```python
from build123d import *

# Parameters (mm, degrees)
EXTRUDE_1_DEPTH        = 10
EXTRUDE_2_DEPTH        = 13.2
SKETCH_3_R             = 2.8
EXTRUDE_3_DEPTH        = 20.1058285
EXTRUDE_3_DEPTH_BACK   = 4
SKETCH_4_R             = 2.8
EXTRUDE_4_DEPTH        = 20.1058285
EXTRUDE_4_DEPTH_BACK   = 4.1058285
SKETCH_5_R             = 2.8
EXTRUDE_5_DEPTH        = 20.1058285
EXTRUDE_5_DEPTH_BACK   = 4.1058285
HOLE_WIZARD_M4_1_D     = 3.3
HOLE_WIZARD_M4_1_DEPTH = 10.1
HOLE_WIZARD_M4_1_TIP   = 0.991420021


with BuildPart() as part:
    # Sketch 1 → Extrude 1 (new body)
    with BuildSketch(Plane.XY):
        Polygon((0, -36.405628463), (31.572352781, 18.279290669), (-31.572352781, 18.279290669), align=None)
    extrude(amount=EXTRUDE_1_DEPTH)

    # Sketch 1_5 → Extrude 2 (add)
    with BuildSketch(Plane.XY):
        Polygon((11.960518161, 2.321180547), (14.039474758, 1.120894396), (16.117440099, -0.078819453), (18.517440099, 4.078102485), (14.360518161, 6.478102485), align=None)
        Polygon((-7.990460401, 9.197522296), (-7.990460401, 12.000572743), (-7.990460401, 13.997522296), (-12.790460401, 13.997522296), (-12.790460401, 9.197522296), align=None)
        Polygon((7.990460401, 14.002477704), (7.990460401, 12.004383545), (7.990460401, 9.202477704), (12.790460401, 9.202477704), (12.790460401, 14.002477704), align=None)
        Polygon((8.131271207, -13.921180547), (6.052314609, -12.720894396), (3.974349269, -11.521180547), (1.574349269, -15.678102485), (5.731271207, -18.078102485), align=None)
        Polygon((-3.97005776, -11.518702843), (-6.395424519, -12.918988994), (-8.126979698, -13.918702843), (-5.726979698, -18.075624781), (-1.57005776, -15.675624781), align=None)
        Polygon((-18.521731608, 4.075624781), (-16.121731608, -0.081297157), (-14.389185172, 0.918988994), (-11.96480967, 2.318702843), (-14.36480967, 6.475624781), align=None)
    extrude(amount=-EXTRUDE_2_DEPTH)

    # Sketch 3 → Extrude 3 (add, two sides)
    with BuildSketch(Plane(origin=(3.9952302, -6.919941695, 0), x_dir=(0.866025404, 0.5, 0), z_dir=(-0.5, 0.866025404, 0))) as extrude_3_sk:
        with Locations((-11.602477704, 13.2)):
            Circle(SKETCH_3_R)
    extrude(amount=EXTRUDE_3_DEPTH)
    extrude(extrude_3_sk.sketch, amount=-EXTRUDE_3_DEPTH_BACK)

    # Sketch 4 → Extrude 4 (add, two sides)
    with BuildSketch(Plane(origin=(-7.990460401, 0, 0), x_dir=(0, 0, -1), z_dir=(1, 0, 0))) as extrude_4_sk:
        with Locations((13.2, 11.602477704)):
            Circle(SKETCH_4_R)
    extrude(amount=EXTRUDE_4_DEPTH)
    extrude(extrude_4_sk.sketch, amount=-EXTRUDE_4_DEPTH_BACK)

    # Sketch 5 → Extrude 5 (add, two sides)
    with BuildSketch(Plane(origin=(3.9952302, 6.919941695, 0), x_dir=(-0.866025404, 0.5, 0), z_dir=(-0.5, -0.866025404, 0))) as extrude_5_sk:
        with Locations((-11.602477704, 13.2)):
            Circle(SKETCH_5_R)
    extrude(amount=EXTRUDE_5_DEPTH)
    extrude(extrude_5_sk.sketch, amount=-EXTRUDE_5_DEPTH_BACK)

    # Hole Wizard M4 _1
    with Locations(Plane.XY.offset(10)):
        with Locations((7.5, 5), (-7.5, 5)):
            Hole(HOLE_WIZARD_M4_1_D / 2, depth=HOLE_WIZARD_M4_1_DEPTH)
            with Locations((0, 0, -(HOLE_WIZARD_M4_1_DEPTH + HOLE_WIZARD_M4_1_TIP / 2))):  # 118° drill point
                Cone(0, HOLE_WIZARD_M4_1_D / 2, HOLE_WIZARD_M4_1_TIP, mode=Mode.SUBTRACT)


solid = part.part
```
Verification items for the finished model (mm, model axes). A direction names the side the tool comes from. Coordinates: 2 decimals unless noted, no trailing zeros. Write each loop counter-clockwise with the first axis right and the second up, starting at its lowest first coordinate (ties: lowest second). Pieces come first, ordered by that corner, then holes. Notation, with made-up numbers: M -3.75,-12.5 L 19.25,-12.5 A17 cw 19.25,12.5 Z; hole C 35.5,67.5 d6. An arc over 180 degrees is marked long. Answer as a JSON object with one key per item and string values. Group by question number.
(1) Cross-section at A-A, the plane z = -8. Record the cut outline in (x, y).
(2) Gauge pin test, flat ends, axial feed: pin 1 (4 mm diameter, centred on y = 10.5, z = -7, fed in from +X); pin 2 (5.5 mm diameter, centred on x = 11, z = -6.5, fed in from +Y); pin 3 (5 mm diameter, centred on y = -4, z = 4.5, fed in from -X); pin 4 (16.5 mm diameter, centred on x = -9.5, y = -20.5, fed in from -Z). Record the tip position at first contact, or that the pin passes through.
(3) Cross-section at B-B, the plane z = 2. Record the cut outline in (x, y).
(4) Cross-section at D-D, the plane x = -24. Record the cut outline in (y, z).
(5) Release check for a two-part mould opening along X. For faces 1 (the face through (-16.007, -8.68, 4.93)), 2 (the face through (-10, 13.998, -7)), 3 (the face through (-3.9, -16.4, -13.2)) record: +X half, -X half, draft (parallel to the pull), parting line (faces both ways), or undercut.
(6) Tool access check on faces 4 (the face through (0, 3, 0)), 5 (the face through (-16, 5, -13.2)), 6 (the face through (16.47, 5.26, -6.51)), 7 (the face through (3.62, -16.86, -6.51)). Record the directions out of +Z, -Z, +X, -X, +Y, -Y that give a thin tool (end or side, any length) a straight path to the whole face; none if there is none.
(7) Material ranges on line 1 (Z direction, x = -13.5, y = 0); line 2 (X direction, y = 9.5, z = -2); line 3 (Z direction, x = -6.5, y = 7), recorded low to high.
(8) Cross-section at C-C, the plane y = 5. State how many separate pieces and enclosed holes the cut face has, and give its area (3 significant figures).
Reply:
{
 "1": {"outline": "M -18.52,4.08 L -16.12,-0.08 L -11.96,2.32 L -14.36,6.48 Z; M -12.79,9.2 L -7.99,9.2 L -7.99,14 L -12.79,14 Z; M -8.13,-13.92 L -5.73,-18.08 L -1.57,-15.68 L -3.97,-11.52 Z; M 1.57,-15.68 L 5.73,-18.08 L 8.13,-13.92 L 3.97,-11.52 Z; M 7.99,9.2 L 12.79,9.2 L 12.79,14 L 7.99,14 Z; M 11.96,2.32 L 16.12,-0.08 L 18.52,4.08 L 14.36,6.48 Z"},
 "2": {"pin 1": "x = 12.79", "pin 2": "y = 14", "pin 3": "x = -20.15", "pin 4": "z = -16"},
 "3": {"outline": "M -31.57,18.28 L 0,-36.41 L 31.57,18.28 Z; hole C -7.5,5 d3.3; hole C 7.5,5 d3.3"},
 "4": {"outline": "M 5.16,0 L 18.28,0 L 18.28,10 L 5.16,10 Z"},
 "5": {"face 1": "-X half", "face 2": "draft", "face 3": "undercut"},
 "6": {"face 4": "none", "face 5": "-Z, -X, +Y", "face 6": "-Z, +X, +Y", "face 7": "-Z, -Y"},
 "7": {"line 1": "-16 to -10.4, 0 to 10", "line 2": "-12.79 to -7.99, 7.99 to 12.79", "line 3": "0 to 10"},
 "8": {"separate pieces": "3", "enclosed holes": "0", "area": "513 mm²"}
}
